Autodesk Inventor part; units mm, degrees
ref_plane "YZ Plane" through (0, 0, 0) normal (1, 0, 0) x (0, 1, 0)
ref_plane "XZ Plane" through (0, 0, 0) normal (0, 1, 0) x (-1, 0, 0)
ref_plane "XY Plane" through (0, 0, 0) normal (0, 0, 1) x (1, 0, 0)
sketch "Sketch2" plane through (0, 0, 0) normal (0, 1, 0) x (-1, 0, 0)
  arc A0 (2, 14) -> (0, 12) centre (2, 12) ccw
  arc A1 (6.0742, 13.1179) -> (35.0957, 13.1179) centre (20.5849, 22.9) ccw
  line L0 (36.754, 14) -> (55.754, 14)
  arc A2 (69.5, 14) -> (57.6905, 15.5) centre (63.5, 14) ccw
  circle A3 centre (63.5, 14) radius 1.5
  arc A4 (55.754, 14) -> (57.6905, 15.5) centre (55.754, 16) ccw
  arc A5 (36.754, 14) -> (35.0957, 13.1179) centre (36.754, 12) ccw
  arc A6 (6.0742, 13.1179) -> (4.4158, 14) centre (4.4158, 12) ccw
  arc A7 (57.3882, 12.2181) -> (55.2287, 14) centre (55.2287, 11.8005) ccw
  line L1 (0, 12) -> (0, 0)
  line L2 (0, 0) -> (69.5, 0)
  line L3 (69.5, 14) -> (69.5, 0)
  arc A8 (57.3882, 12.2181) -> (69.5, 11.7415) centre (63.5, 13.4) ccw
  line L4 (4.4158, 14) -> (2, 14)
  point P0 (0, 0)
  point P1 (20.5849, 5.4)
  dimension "d3" = 2
  dimension "d17" = 3
  dimension "d18" = 2
  dimension "d137" = 2.1995
  dimension "d140" = 12
  dimension "d141" = 69.5
  dimension "d142" = 14
  dimension "d143" = 6
  dimension "d144" = 17.5
  dimension "d145" = 19
  dimension "d146" = 5.4
  dimension "d147" = 6.225
  dimension "d148" = 13.4
extrude "Extrusion1" add sketch "Sketch2" along normal mid plane 30
extrude "Extrusion2" cut sketch "Sketch2" along normal mid plane 15 contours A8 A7 L0 A4 A2 L3
sketch "Sketch7" plane through (0, -15, 0) normal (0, -1, 0) x (1, 0, 0)
  arc A0 (-4.4158, 14) -> (-6.0742, 13.1179) centre (-4.4158, 12) ccw
  line L0 (-6.0742, 13.1179) -> (-6.0742, 12.1179)
  arc A1 (-35.0957, 13.1179) -> (-6.0742, 13.1179) centre (-20.5849, 22.9) ccw
  line L1 (-35.0957, 13.1179) -> (-35.0957, 12.1179)
  arc A2 (-35.0957, 12.1179) -> (-6.0742, 12.1179) centre (-20.5849, 22.8831) ccw
  point P0 (0, 0)
  point P1 (-6.3389, 0)
  dimension "d59" = 1
  dimension "d60" = 1
extrude "Extrusion10" cut sketch "Sketch7" against normal up to next
fillet "Fillet4" radius 2 1 edges at (-69.5, 0, 11.7415)
sketch "Sketch13" plane through (-55.754, -15, 14) normal (0, 0, 1) x (1, 0, 0)
  circle A0 centre (8.754, 15) radius 4
  line L0 (55.754, 0) -> (55.754, 30)
  line L1 (14.254, 18.1754) -> (14.254, 11.8246)
  line L2 (14.254, 11.8246) -> (8.754, 8.6491)
  line L3 (8.754, 8.6491) -> (3.254, 11.8246)
  line L4 (3.254, 11.8246) -> (3.254, 18.1754)
  line L5 (3.254, 18.1754) -> (8.754, 21.3509)
  line L6 (8.754, 21.3509) -> (14.254, 18.1754)
  line L7 (19, 0) -> (0, 0)
  circle A1 centre (8.754, 26) radius 1.1
  line L8 (8.754, 15) -> (25.6273, 15) construction
  line L9 (9.9232, 23.975) -> (7.5849, 23.975)
  line L10 (7.5849, 23.975) -> (6.4158, 26)
  line L11 (6.4158, 26) -> (7.5849, 28.025)
  line L12 (7.5849, 28.025) -> (9.9232, 28.025)
  line L13 (9.9232, 28.025) -> (11.0923, 26)
  line L14 (11.0923, 26) -> (9.9232, 23.975)
  circle A2 centre (8.754, 4) radius 1.1
  line L15 (9.9232, 6.025) -> (7.5849, 6.025)
  line L16 (7.5849, 6.025) -> (6.4158, 4)
  line L17 (6.4158, 4) -> (7.5849, 1.975)
  line L18 (7.5849, 1.975) -> (9.9232, 1.975)
  line L19 (9.9232, 1.975) -> (11.0923, 4)
  line L20 (11.0923, 4) -> (9.9232, 6.025)
  point P0 (55.754, 15)
  dimension "d99" = 8
  dimension "d106" = 47
  dimension "d131" = 11
  dimension "d132" = 15
  dimension "d159" = 2.2
  dimension "d160" = 11
  dimension "d163" = 4.05
extrude "Extrusion15" cut sketch "Sketch13" against normal up to next contours A0
sketch "Sketch17" plane through (-55.754, -15, 14) normal (0, 0, 1) x (1, 0, 0)
  point P0 (55.754, 15)
sketch "Sketch19" plane through (0, 15, 0) normal (0, 0, -1) x (-1, 0, 0)
  circle A0 centre (47, -15) radius 4
  line L0 (47, -21.4663) -> (41.4, -18.2332)
  line L1 (41.4, -18.2332) -> (41.4, -11.7668)
  line L2 (41.4, -11.7668) -> (47, -8.5337)
  line L3 (47, -8.5337) -> (52.6, -11.7668)
  line L4 (52.6, -11.7668) -> (52.6, -18.2332)
  line L5 (52.6, -18.2332) -> (47, -21.4663)
  point P0 (0, -15)
  dimension "d156" = 11.2
extrude "Extrusion23" cut sketch "Sketch19" against normal blind 4.5
sketch "Sketch20" plane through (0, 15, 0) normal (0, 1, 0) x (1, 0, 0)
  point P0 (0, 0)
extrude "Extrusion24" cut sketch "Sketch13" against normal up to next contours A1 | A2
extrude "Extrusion25" cut sketch "Sketch13" against normal blind 1.7 contours A1 | L9 L10 L11 L12 L13 L14 | A2 | L20 L19 L18 L17 L16 L15
properties part number "Bike_Mount_Right" material "PC/ABS Plastic"
Source: CAD feature listing. Evaluate the final solid. Frame: model axes, mm. A direction names the side the tool comes from. Round coordinates to 2 decimals unless told otherwise and drop trailing zeros. Write each loop counter-clockwise with the first axis right and the second up, starting at its lowest first coordinate (ties: lowest second). Pieces come first, ordered by that corner, then holes. Notation, with made-up numbers: (83, -34) - (116, -34) arc R27 ccw to (116, -13) - close; hole circle Ø11 at (-21.75, -17.5). An arc over 180 degrees is marked (long way). Use CSV: the item, a comma, the result in double quotes. Start each with the question number.
(1) Material intervals for probe 1 along Y at (x, z) = (-47, 2.5); probe 2 along Z at (x, y) = (-63.5, 13.25); probe 3 along X at (y, z) = (10.5, 13.25), sorted ascending. Write a range as [from, to].
(2) Cut plane D-D, the plane x = -32.5. Return loops of the section in (y, z).
(3) Mould query, pull axis X, two halves, no side actions, for faces 5 (the face through (-35.8, -0.21, 13.76)), 6 (the face through (-69.5, 0, 6)), 7 (the face through (-42, -15, 8)). Classes: pulls with the +X half, pulls with the -X half, needs draft (parallel to the pull), parting line crosses it, or undercut.
(4) Set-up query: faces 1 (the face through (-56.99, -11.3, 14.43)), 2 (the face through (-47, 13.025, 13)), 3 (the face through (-56.61, -0.11, 13.51)), 4 (the face through (-41.4, 0, 2)). Return all of +Z, -Z, +X, -X, +Y, -Y with unobstructed straight access to the full face (end or side cutting, diameter ignored); none if empty.
(5) Cut plane C-C, the plane y = 0. Return loops of the section in (x, z) (1 decimal).
(6) Cut plane A-A, the plane x = -63.5. Return loops of the section in (y, z), and give its area (3 significant figures).
(7) Cut plane B-B, the plane z = 10.75. Return loops of the section in (x, y), and give its area (3 significant figures).
(8) First-contact query: pin 1 Ø4 at (y, z) = (-1, 14.5) entering from -X; pin 2 Ø2.5 at (x, z) = (-63.5, 14) entering from +Y; pin 3 Ø1 at (x, y) = (-32.5, 7.5) entering from +Z; pin 4 Ø1.9 at (x, y) = (-3, -4.5) entering from +Z. Flat tips, straight axial feed; report the tip coordinate or a pass-through.
Geometry says:
1,probe 1,"[-15, -12.1], [-9.9, -6.47], [6.47, 9.9], [12.1, 15]"
1,probe 2,"[0, 12.5], [15.5, 20]"
1,probe 3,"[-69.5, -64.8], [-62.2, -49.05], [-44.95, -35.19], [-5.98, -0.44]"
2,outline,"(-15, 0) - (15, 0) - (15, 9.3) - (-15, 9.3) - close"
3,face 5,"undercut"
3,face 6,"pulls with the -X half"
3,face 7,"needs draft"
4,face 1,"+Z, +X, +Y, -Y"
4,face 2,"+Z"
4,face 3,"+Z, -X"
4,face 4,"-Z"
5,outline,"(-69.5, 0) - (-52.6, 0) - (-52.6, 4.5) - (-51, 4.5) - (-51, 14) - (-55.2, 14) arc R2.2 ccw to (-57.4, 12.2) arc R6.2 cw to (-66.5, 8) arc R2 ccw to (-69.5, 6.2) - close; (-43, 4.5) - (-41.4, 4.5) - (-41.4, 0) - (0, 0) - (0, 12) arc R2 ccw to (-2, 14) - (-4.4, 14) arc R2 ccw to (-6.1, 13.1) - (-6.1, 12.1) arc R18.1 cw to (-35.1, 12.1) - (-35.1, 13.1) arc R2 ccw to (-36.8, 14) - (-43, 14) - close"
6,outline,"(-15, 0) - (15, 0) - (15, 12.5) - (7.5, 12.5) - (7.5, 7.17) - (-7.5, 7.17) - (-7.5, 12.5) - (-15, 12.5) - close; (-15, 15.5) - (-7.5, 15.5) - (-7.5, 20) - (-15, 20) - close; (7.5, 15.5) - (15, 15.5) - (15, 20) - (7.5, 20) - close"
6,area,"363 mm²"
7,outline,"(-69.5, -15) - (-33.97, -15) - (-33.97, 15) - (-69.5, 15) - (-69.5, 7.5) - (-57.87, 7.5) - (-57.87, -7.5) - (-69.5, -7.5) - close; (-7.2, -15) - (0, -15) - (0, 15) - (-7.2, 15) - close; hole circle Ø8 at (-47, 0); hole circle Ø2.2 at (-47, -11); hole circle Ø2.2 at (-47, 11)"
7,area,"1,050 mm²"
8,pin 1,"x = -57.31"
8,pin 2,"through"
8,pin 3,"z = 9.76"
8,pin 4,"z = 14"
